Input: dimensioned drawing with shaded views. Units: mm. Origin: part minimum x, y, z. Give positions to 0.01 mm unless a question says otherwise; leave off trailing zeros. Order: outer loops, then holes, each group sorted by start corner. A loop starts at its lowest first (then second) coordinate and runs counter-clockwise, first axis right, second up.
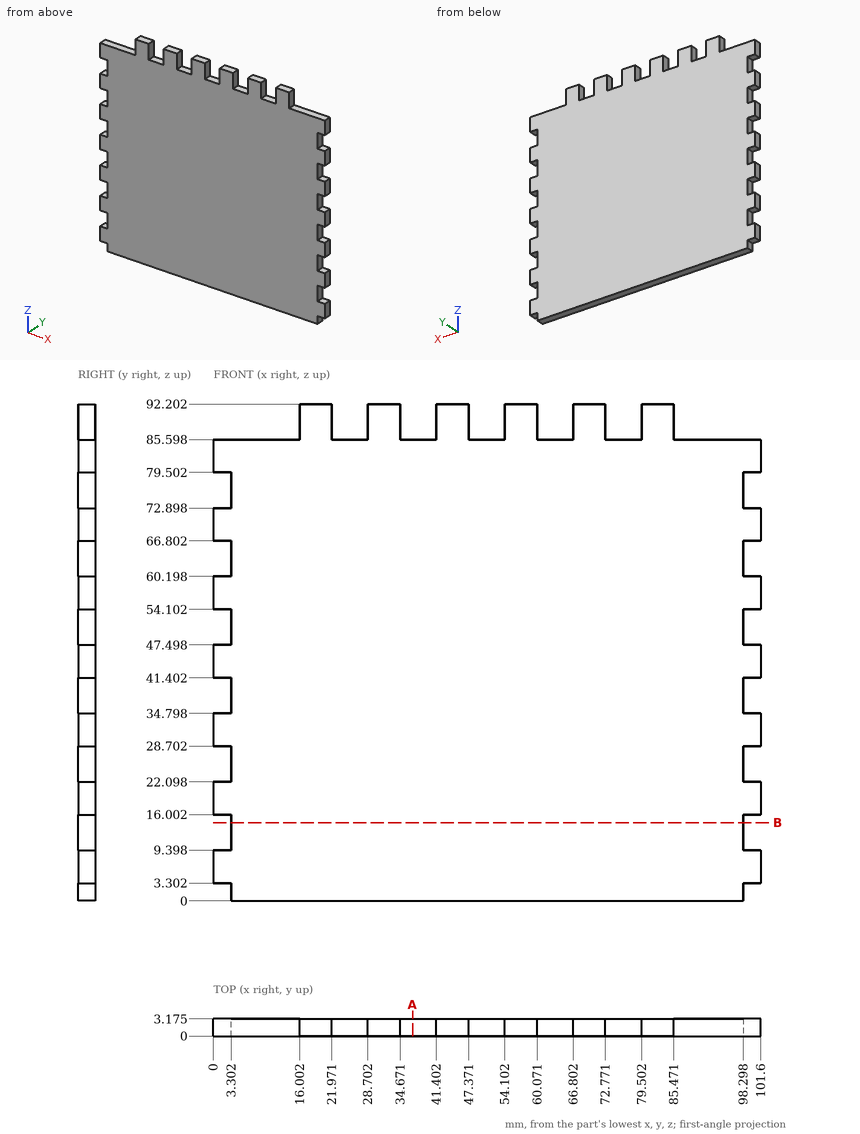
1) Material intervals for L1, parallel to Z at x = 51.5, y = 2.05; L2, parallel to X at y = 0.65, z = 74, sorted ascending.
Report:
L1: z = 0 to 85.6
L2: x = 3.3 to 98.3
2) Section query A-A, the plane x = 37. Return the cut outline in (y, z) (3 decimals).
Report:
outline: (0, 0) - (3.175, 0) - (3.175, 85.598) - (0, 85.598) - close
3) Section query B-B, the plane z = 14.5. Return the cut outline in (x, y) (3 decimals), and give its area (3 significant figures).
Report:
outline: (3.302, 0) - (98.298, 0) - (98.298, 3.175) - (3.302, 3.175) - close
area: 302 mm2
4) Pin query (flat end, axial travel): pin 1 (1 mm diameter, centred on x = 1, y = 1.5, fed in from +Z); pin 2 (1.6 mm diameter, centred on y = 1.5, z = 50.5, fed in from +X); pin 3 (1.6 mm diameter, centred on y = 2, z = 89.5, fed in from -X). Return the tip coordinate at first contact, or that it passes through.
Report:
pin 1: stops at z = 85.6
pin 2: stops at x = 98.3
pin 3: stops at x = 16
